from build123d import *

# Parameters (mm, degrees)
SKETCH_1_W                          = 40
SKETCH_1_H                          = 9
EXTRUDE_1_DEPTH                     = 4.3
SKETCH_2_W                          = 0.85
SKETCH_2_H                          = 0.9
EXTRUDE_2_DEPTH                     = 9
CHAMFER_1_SIZE                      = 0.09
PATTERN_LINEAR_10_COUNT             = 7
PATTERN_LINEAR_10_PITCH             = 1.7
CHAMFER_1_OF_PATTERN_LINEAR_10_SIZE = 0.09
MIRROR_START                        = -4.5
MIRROR_3_DEPTH                      = 9
SKETCH_4_R                          = 2
CUT_EXTRUDE_1_DEPTH                 = 21.946121359
CHAMFER_2_SIZE                      = 0.5
CHAMFER_3_SIZE                      = 0.1


# Read off the part's stored shape, not the designer's step: 鏡射3
with BuildPart() as part:
    # 草圖1 → 填料-伸長1 (new body)
    with BuildSketch(Plane(origin=(0, 0, 0), x_dir=(1, 0, 0), z_dir=(0, 1, 0))):
        Rectangle(SKETCH_1_W, SKETCH_1_H)
    extrude(amount=EXTRUDE_1_DEPTH)

    # 草圖2 → 填料-伸長2 (add)
    with BuildSketch(Plane.XY.offset(4.5)):
        with Locations((-19.575, 4.75)):
            Rectangle(SKETCH_2_W, SKETCH_2_H)
    extrude_2 = extrude(amount=-EXTRUDE_2_DEPTH)

    # 導角1
    chamfer_1_edges = [part.edges().sort_by_distance(p)[0] for p in [
        (-20, 5.2, 0),
        (-19.15, 5.2, 0),
    ]]
    chamfer(chamfer_1_edges, length=CHAMFER_1_SIZE)

    # 直線複製排列10: 填料-伸長2 ×7
    with Locations(*[(i * PATTERN_LINEAR_10_PITCH, 0, 0) for i in range(1, PATTERN_LINEAR_10_COUNT)]):
        add(extrude_2)

    # 導角1 of 直線複製排列10
    chamfer_1_of_pattern_linear_10_edges = [part.edges().sort_by_distance(p)[0] for p in [
        (-18.3, 5.2, 0),
        (-17.45, 5.2, 0),
        (-16.6, 5.2, 0),
        (-15.75, 5.2, 0),
        (-14.9, 5.2, 0),
        (-14.05, 5.2, 0),
        (-13.2, 5.2, 0),
        (-12.35, 5.2, 0),
        (-11.5, 5.2, 0),
        (-10.65, 5.2, 0),
        (-9.8, 5.2, 0),
        (-8.95, 5.2, 0),
    ]]
    chamfer(chamfer_1_of_pattern_linear_10_edges, length=CHAMFER_1_OF_PATTERN_LINEAR_10_SIZE)

    # 鏡射3 outline → 鏡射3 (add)
    with BuildSketch(Plane.XY.offset(MIRROR_START)):
        Polygon((8.95, 4.3), (9.8, 4.3), (9.8, 5.11), (9.71, 5.2), (9.04, 5.2), (8.95, 5.11), align=None)
        Polygon((10.65, 4.3), (11.5, 4.3), (11.5, 5.11), (11.41, 5.2), (10.74, 5.2), (10.65, 5.11), align=None)
        Polygon((12.35, 4.3), (13.2, 4.3), (13.2, 5.11), (13.11, 5.2), (12.44, 5.2), (12.35, 5.11), align=None)
        Polygon((14.05, 4.3), (14.9, 4.3), (14.9, 5.11), (14.81, 5.2), (14.14, 5.2), (14.05, 5.11), align=None)
        Polygon((15.75, 4.3), (16.6, 4.3), (16.6, 5.11), (16.51, 5.2), (15.84, 5.2), (15.75, 5.11), align=None)
        Polygon((17.45, 4.3), (18.3, 4.3), (18.3, 5.11), (18.21, 5.2), (17.54, 5.2), (17.45, 5.11), align=None)
        Polygon((20, 4.3), (20, 5.11), (19.91, 5.2), (19.24, 5.2), (19.15, 5.11), (19.15, 4.3), align=None)
    extrude(amount=MIRROR_3_DEPTH)

    # 草圖4 → 除料-伸長1 (cut, through all)
    with BuildSketch(Plane(origin=(0, 4.3, 0), x_dir=(1, 0, 0), z_dir=(0, 1, 0))):
        with Locations(Location((0, 0, 0), (0, 0, 270))):
            Circle(SKETCH_4_R)
    extrude(amount=-CUT_EXTRUDE_1_DEPTH, mode=Mode.SUBTRACT)

    # 導角2
    chamfer_2_edges = [part.edges().sort_by_distance(p)[0] for p in [
        (0, 4.3, -2),
    ]]
    chamfer(chamfer_2_edges, length=CHAMFER_2_SIZE)

    # 導角3
    chamfer_3_edges = [part.edges().sort_by_distance(p)[0] for p in [
        (0, 4.3, -4.5),
        (0, 4.3, 4.5),
    ]]
    chamfer(chamfer_3_edges, length=CHAMFER_3_SIZE)


solid = part.part
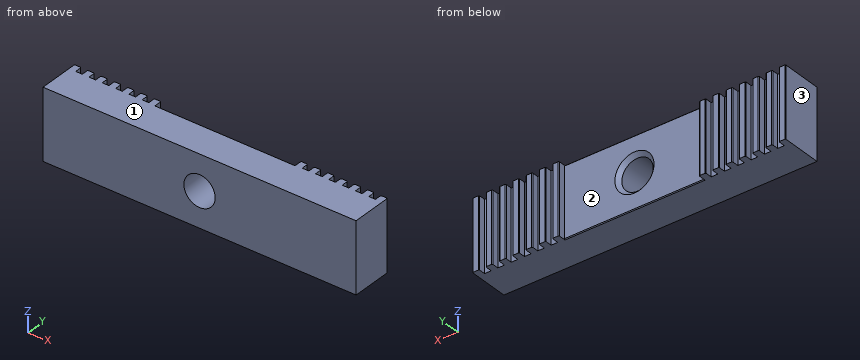
Geometry: final body of the model. Coordinates: model frame, mm. Face numbers are marked on the shaded views. Coordinates: 2 decimals unless noted, no trailing zeros. Order: outer loops, then holes, each group sorted by start corner. A loop starts at its lowest first (then second) coordinate and runs counter-clockwise, first axis right, second up.
1) Section A-A (x = 0). Return loops of the section in (y, z).
Result sheet:
outline: (0, -4.5) - (4.2, -4.5) - (4.3, -4.4) - (4.3, -2.5) - (3.8, -2) - (0, -2) - close; (0, 2) - (3.8, 2) - (4.3, 2.5) - (4.3, 4.4) - (4.2, 4.5) - (0, 4.5) - close
2) Draft query along X for the marked faces 1, 2 and 3. Return one class per face: released by +X, released by -X, zero draft, split by the parting line, or undercut.
Result sheet:
face 1: zero draft
face 2: undercut
face 3: released by -X
3) Section C-C (x = 8). Return loops of the section in (y, z), then the cut area to 3 significant figures.
Result sheet:
outline: (0, -4.5) - (4.2, -4.5) - (4.3, -4.4) - (4.3, 4.4) - (4.2, 4.5) - (0, 4.5) - close
area: 38.7 mm2
4) First-contact query: P1, Ø0.7, axis at x = -11.5, z = -1, coming from the +Y side. Flat tip, straight axial feed; report the tip coordinate or a pass-through.
Result sheet:
P1: stops at y = 5.2
5) Section B-B (y = 0.9). Return loops of the section in (x, z).
Result sheet:
outline: (-20, -4.5) - (20, -4.5) - (20, 4.5) - (-20, 4.5) - close; hole circle Ø4 at (0, 0)
6) Ray query, probe 1 along X at (y, z) = (0.8, 0); probe 2 along Y at (x, z) = (10, -2.25); probe 3 along Z at (x, y) = (1, 2.25). Return the intervals inside material, ascending.
Result sheet:
probe 1: x = -20 to -2, 2 to 20
probe 2: y = 0 to 4.3
probe 3: z = -4.5 to -1.73, 1.73 to 4.5
